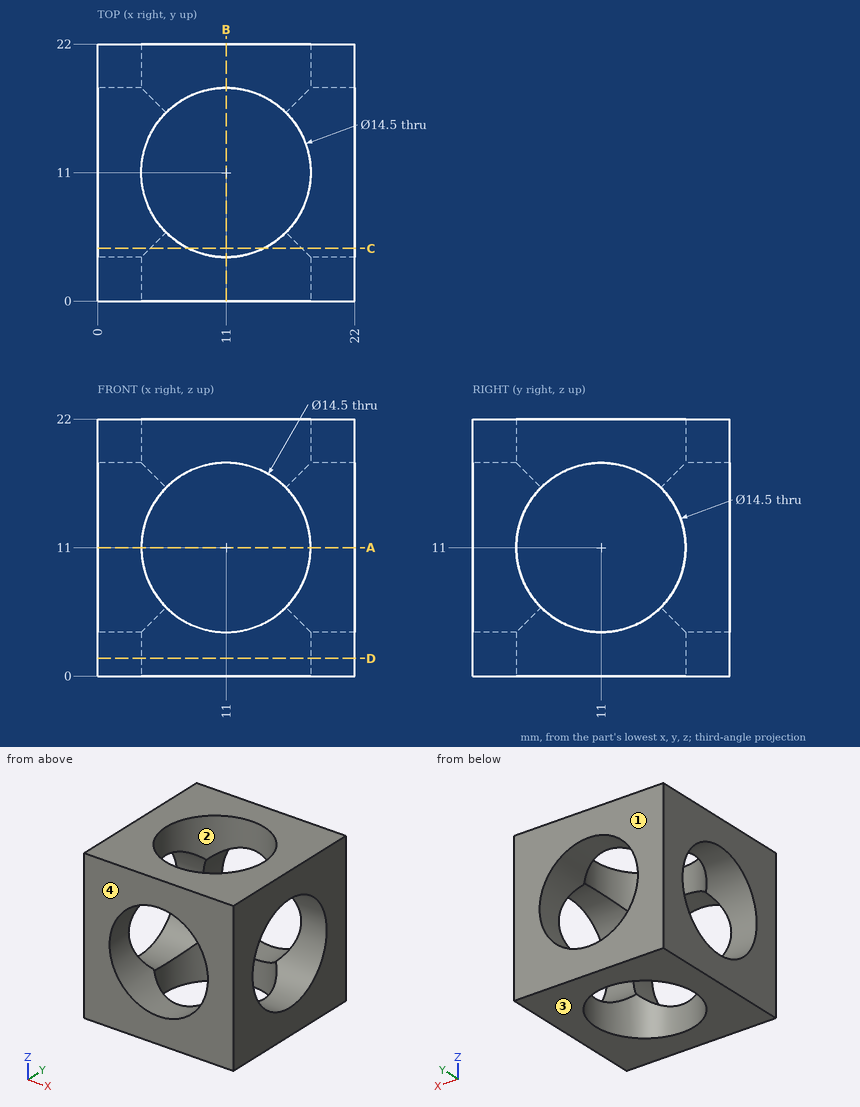
Source: three-view drawing plus pictorial views. Frame: mm from the lowest corner of the part. Round coordinates to 2 decimals unless told otherwise and drop trailing zeros. Loops run counter-clockwise (first coordinate to the right, second up) from the corner with the lowest first, then second, coordinate; pieces in that order, holes last. Notation, with made-up numbers: M 9,86.25 L 18,86.25 A17 ccw 18,100.25 Z; hole C 12,26.5 d5. An arc over 180 degrees is marked long. Put each result on its own line as item: value.
(1) First-contact query: pin 1 (1 mm diameter, centred on x = 5.5, z = 8, fed in from -Y). Flat tip, straight axial feed; report the tip coordinate or a pass-through.
Solutions:
pin 1: through
(2) Section A-A, the plane z = 11. Return loops of the section in (x, y).
Solutions:
outline: M 0,0 L 3.75,0 L 3.75,3.75 L 0,3.75 Z; M 0,18.25 L 3.75,18.25 L 3.75,22 L 0,22 Z; M 18.25,0 L 22,0 L 22,3.75 L 18.25,3.75 Z; M 18.25,18.25 L 22,18.25 L 22,22 L 18.25,22 Z
(3) Section D-D, the plane z = 1.5. Return loops of the section in (x, y).
Solutions:
outline: M 0,0 L 22,0 L 22,22 L 0,22 Z; hole C 11,11 d14.5
(4) Section C-C, the plane y = 4.5. Return loops of the section in (x, z), and give its area (3 significant figures).
Solutions:
outline: M 0,0 L 7.79,0 L 7.79,4.5 A7.25 cw 4.5,7.79 L 0,7.79 Z; M 0,14.21 L 4.5,14.21 A7.25 cw 7.79,17.5 L 7.79,22 L 0,22 Z; M 14.21,0 L 22,0 L 22,7.79 L 17.5,7.79 A7.25 cw 14.21,4.5 Z; M 14.21,17.5 A7.25 cw 17.5,14.21 L 22,14.21 L 22,22 L 14.21,22 Z
area: 216 mm²
(5) Pull-direction query (Y, two-part tool) for the marked faces 1, 2, 3 and 4; classes: released by +Y, released by -Y, zero draft, split by the parting line, or undercut.
Solutions:
face 1: released by +Y
face 2: undercut
face 3: zero draft
face 4: released by -Y
(6) Ray query, line 1 (X direction, y = 11, z = 18.9). Return the intervals inside material, ascending. Write a range as [from, to].
Solutions:
line 1: [0, 3.75], [18.25, 22]
